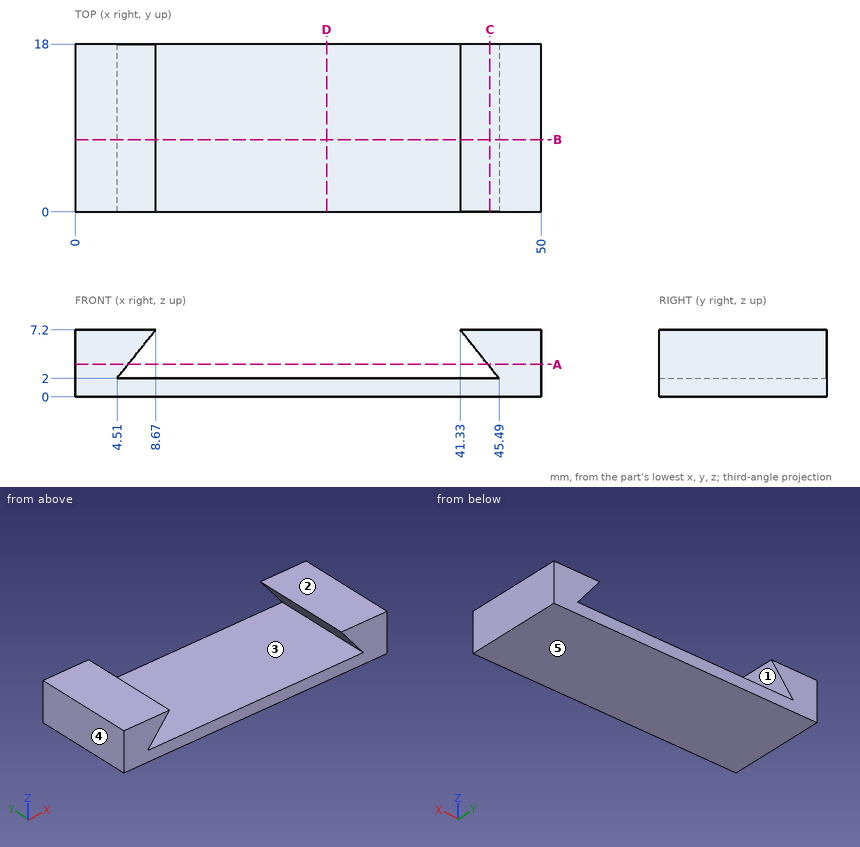
Drawing for the job (mm, zero at the part's lowest x, y, z). A direction names the side the tool comes from. Give positions to 0.01 mm unless a question says otherwise; leave off trailing zeros. Write each loop counter-clockwise with the first axis right and the second up, starting at its lowest first coordinate (ties: lowest second). Pieces come first, ordered by that corner, then holes. Notation, with made-up numbers: (-4, 4) - (51, 4) arc R27 cw to (51, 25) - close; hole circle Ø7 at (29, 74). An arc over 180 degrees is marked (long way). Answer as CSV lines item,"result".
Q1. Drill centre lines: line 1 (Z direction, x = 29, y = 9.25); line 2 (X direction, y = 9.5, z = 4.75); line 3 (Z direction, x = 43, y = 3.5). Where is each one in solid material? Low to high. Write a range as from..to.
Result set:
line 1,"0..2"
line 2,"0..6.71, 43.29..50"
line 3,"0..2, 5.11..7.2"
Q2. Band-saw the part on C-C (x = 44.5). Give the cut face in (y, z).
Result set:
outline,"(0, 0) - (18, 0) - (18, 2) - (0, 2) - close; (0, 3.24) - (18, 3.24) - (18, 7.2) - (0, 7.2) - close"
Q3. Flat gauge pin, fed straight in: pin 1 Ø8 at (x, y) = (26, 14) entering from +Z. Where does the tip first touch, or does it go through?
Result set:
pin 1,"z = 2"
Q4. Pull direction X, two halves, no side cores. Call the marked faces 3, 4 and 5: released by +X, released by -X, zero draft, split by the parting line, or undercut.
Result set:
face 3,"undercut"
face 4,"released by -X"
face 5,"zero draft"
Q5. Band-saw the part on B-B (y = 7.75). Give the cut face in (x, z), and give its area (3 significant figures).
Result set:
outline,"(0, 0) - (50, 0) - (50, 7.2) - (41.33, 7.2) - (45.49, 2) - (4.51, 2) - (8.67, 7.2) - (0, 7.2) - close"
area,"169 mm²"
Q6. 3-axis set-ups, long thin cutter, end or side, ignore diameter. For the marked faces 1 and 2: which of +Z, -Z, +X, -X, +Y, -Y reach the whole face in a straight line?
Result set:
face 1,"+Y, -Y"
face 2,"+Z, +X, -X, +Y, -Y"
Q7. Band-saw the part on A-A (z = 3.5). Give the cut face in (x, y).
Result set:
outline,"(0, 0) - (5.71, 0) - (5.71, 18) - (0, 18) - close; (44.29, 0) - (50, 0) - (50, 18) - (44.29, 18) - close"
Q8. Band-saw the part on D-D (x = 27). Give the cut face in (y, z).
Result set:
outline,"(0, 0) - (18, 0) - (18, 2) - (0, 2) - close"
